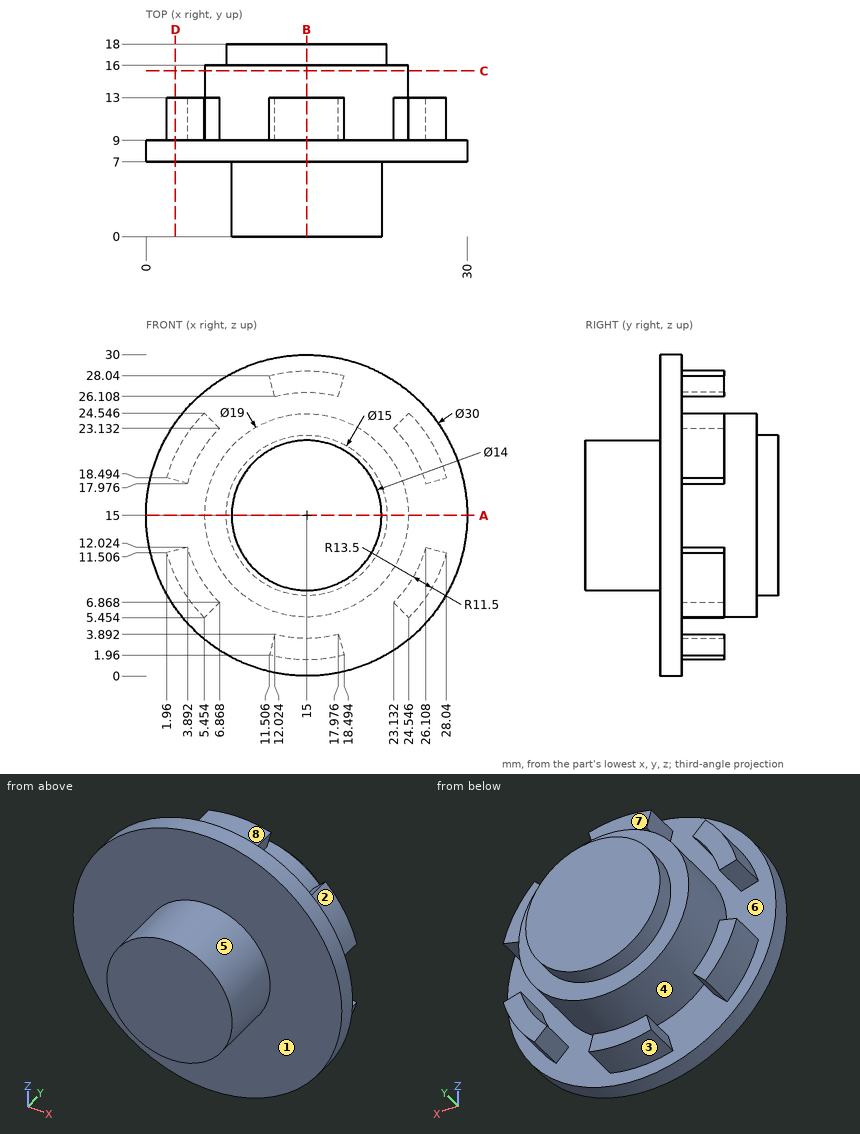
The figure shows three views and two pictorial views of one solid part (mm, origin at its lowest corner). Answer the questions. A direction names the side the tool comes from. Give positions to 0.01 mm unless a question says otherwise; leave off trailing zeros. Order: outer loops, then holes, each group sorted by start corner. A loop starts at its lowest first (then second) coordinate and runs counter-clockwise, first axis right, second up. Notation, with made-up numbers: (41, 28) -> (77, 28) arc R13 cw to (77, 47) -> close; hole circle Ø8 at (-27.75, 24.25). An arc over 180 degrees is marked (long way). Answer as CSV lines item,"result". Start each with the question number.
Q1. Which of the six approach directions +Z, -Z, +X, -X, +Y, -Y give full straight-line access (tool end or side, diameter ignored) to the marked faces 1, 2, 3 and 4?
Q2. A cutting plane is placed at D-D (x = 2.75). Determine the outline of the cut face in (y, z).
Q3. A cutting plane is placed at A-A (z = 15). Determine the outline of the cut face in (x, y), then the cut area to 3 significant figures.
Q4. A cutting plane is placed at B-B (x = 15). Determine the outline of the cut face in (y, z).
Q5. Given pin 1 (1 mm diameter, centred on x = 24, y = 14.5, fed in from +Z) (1 decimal); pin 2 (2.5 mm diameter, centred on x = 5, z = 9, fed in from +Y); pin 3 (4 mm diameter, centred on x = 24.5, z = 21, fed in from +Y), each flat-ended and moving along its own axis, determine where each tip first touches the part or whether it passes through.
Q6. A cutting plane is placed at C-C (y = 15.5). Determine the outline of the cut face in (x, z).
Q7. Find the intervals of material crossed by L1, parallel to X at y = 10.25, z = 23.5 (1 decimal); L2, parallel to Y at x = 11, z = 21.25; L3, parallel to Z at x = 5.25, y = 11.75 (1 decimal), in increasing order.
Q8. Determine the mould class of the marked faces 5, 6, 7 and 8 for opening direction Z: pulls with the +Z half, pulls with the -Z half, needs draft (parallel to the pull), parting line crosses it, or undercut.
Results found:
1,face 1,"-Y"
1,face 2,"+Z, +X, +Y"
1,face 3,"-Z, +Y"
1,face 4,"+Y"
2,outline,"(7, 6.34) -> (9, 6.34) -> (9, 9.33) -> (13, 9.33) -> (13, 11.72) -> (9, 11.72) -> (9, 18.28) -> (13, 18.28) -> (13, 20.67) -> (9, 20.67) -> (9, 23.66) -> (7, 23.66) -> close"
3,outline,"(0, 7) -> (8, 7) -> (8, 0) -> (22, 0) -> (22, 7) -> (30, 7) -> (30, 9) -> (24.5, 9) -> (24.5, 16) -> (22.5, 16) -> (22.5, 18) -> (7.5, 18) -> (7.5, 16) -> (5.5, 16) -> (5.5, 9) -> (0, 9) -> close"
3,area,"321 mm2"
4,outline,"(0, 8) -> (7, 8) -> (7, 0) -> (9, 0) -> (9, 1.5) -> (13, 1.5) -> (13, 3.5) -> (9, 3.5) -> (9, 5.5) -> (16, 5.5) -> (16, 7.5) -> (18, 7.5) -> (18, 22.5) -> (16, 22.5) -> (16, 24.5) -> (9, 24.5) -> (9, 26.5) -> (13, 26.5) -> (13, 28.5) -> (9, 28.5) -> (9, 30) -> (7, 30) -> (7, 22) -> (0, 22) -> close"
5,pin 1,"z = 19.2"
5,pin 2,"y = 13"
5,pin 3,"y = 16"
6,outline,"circle Ø19 at (15, 15)"
7,L1,"4.5 to 6.5, 10.8 to 19.2, 23.5 to 25.5"
7,L2,"7 to 18"
7,L3,"5.7 to 8.9, 21.1 to 24.3"
8,face 5,"parting line crosses it"
8,face 6,"undercut"
8,face 7,"needs draft"
8,face 8,"pulls with the +Z half"
